Here's the drawing with two shaded views (mm, measured from the low corner). I have some questions. Coordinates: 2 decimals unless noted, no trailing zeros. Order: outer loops, then holes, each group sorted by start corner. A loop starts at its lowest first (then second) coordinate and runs counter-clockwise, first axis right, second up. Notation, with made-up numbers: (73, -21.5) - (92, -21.5) arc R25 cw to (92, -4.5) - close; hole circle Ø3 at (16.25, 47.25). An arc over 180 degrees is marked (long way). Answer as CSV lines item,"result". Start each with the question number.
1. I want a section at A-A, the plane x = 3.35. List the corners of the cut face in (y, z) for me, and give its area (3 significant figures).
2. I want a section at C-C, the plane z = 3.35. List the corners of the cut face in (x, y) for me, and give its area (3 significant figures).
3. Thinking about a two-plate mould opening in X: for the marked faces 1, 2 and 3, which applies, released by +X, released by -X, zero draft, split by the parting line, or undercut?
4. I need wall thicknesses on probe 1 along Z at (x, y) = (3.35, 0.25); probe 2 along Z at (x, y) = (4, 0.2); probe 3 along X at (y, z) = (0.6, 3). Which ranges of each line are inside material? Lowest first, please.
5. I want a section at B-B, the plane y = 0.1. List the corners of the cut face in (x, z) for me, and give its area (3 significant figures).
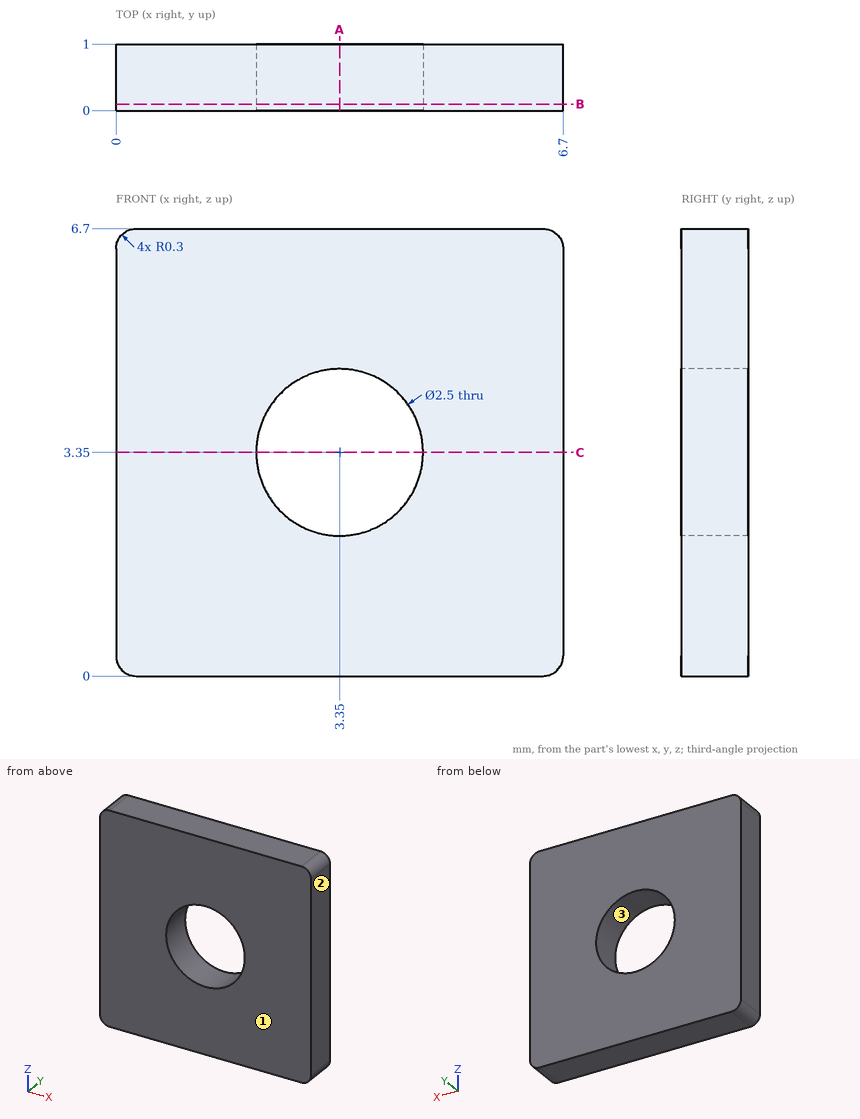
Solved:
1,outline,"(0, 0) - (1, 0) - (1, 2.1) - (0, 2.1) - close; (0, 4.6) - (1, 4.6) - (1, 6.7) - (0, 6.7) - close"
1,area,"4.20 mm2"
2,outline,"(0, 0) - (2.1, 0) - (2.1, 1) - (0, 1) - close; (4.6, 0) - (6.7, 0) - (6.7, 1) - (4.6, 1) - close"
2,area,"4.20 mm2"
3,face 1,"zero draft"
3,face 2,"released by +X"
3,face 3,"undercut"
4,probe 1,"z = 0 to 2.1, 4.6 to 6.7"
4,probe 2,"z = 0 to 2.28, 4.42 to 6.7"
4,probe 3,"x = 0 to 2.15, 4.55 to 6.7"
5,outline,"(0, 0.3) arc R0.3 ccw to (0.3, 0) - (6.4, 0) arc R0.3 ccw to (6.7, 0.3) - (6.7, 6.4) arc R0.3 ccw to (6.4, 6.7) - (0.3, 6.7) arc R0.3 ccw to (0, 6.4) - close; hole circle Ø2.5 at (3.35, 3.35)"
5,area,"39.9 mm2"
